Source: CAD feature listing. Evaluate the final solid. Frame: model axes, mm. Round coordinates to 2 decimals unless told otherwise and drop trailing zeros. Write each loop counter-clockwise with the first axis right and the second up, starting at its lowest first coordinate (ties: lowest second). Pieces come first, ordered by that corner, then holes. Notation, with made-up numbers: M 86.5,74 L 131.5,74 A20 ccw 131.5,101 Z; hole C 79.25,-22.5 d7. An arc over 180 degrees is marked long. Use a Markdown table: item, result.
```python
from build123d import *

# Parameters (mm, degrees)
PAD_DEPTH = 10


with BuildPart() as part:
    # Sketch → Pad (new body)
    with BuildSketch(Plane.XY):
        with BuildLine():
            Line((2.012226, 0), (22.012226, 0))
            ThreePointArc((22.012226, 0), (25.943926, 1.628563), (27.572489, 5.560263))
            Line((27.572489, 5.560263), (27.572489, 423.618953))
            ThreePointArc((46.701722, 450.938329), (32.830223, 440.294353), (27.572489, 423.618953))
            Line((46.701722, 450.938329), (760.532733, 710.751569))
            Line((760.532733, 713.751569), (760.532733, 710.751569))
            Line((24.572489, 455.938329), (760.532733, 713.751569))
            Line((24.572489, 3), (24.572489, 455.938329))
            Line((-1.804961, 3), (24.572489, 3))
            Line((-1.804961, -7), (-1.804961, 3))
            Line((21.983993, -7), (-1.804961, -7))
            Line((21.983993, -4), (21.983993, -7))
            Line((1.983993, -4), (21.983993, -4))
            ThreePointArc((0, -2.016007), (0.581098, -3.418902), (1.983993, -4))
            Line((0, -2.012226), (0, -2.016007))
            ThreePointArc((2.012226, 0), (0.589367, -0.589367), (0, -2.012226))
        make_face()
    extrude(amount=PAD_DEPTH)


solid = part.part
```
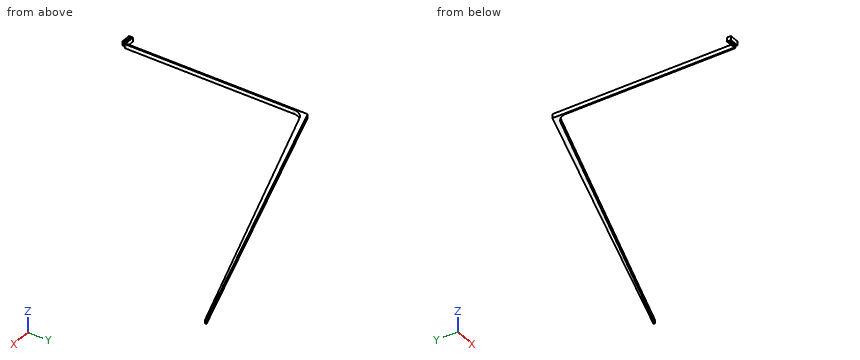
Q1. Line query: L1, parallel to X at y = 299, z = 7.25; L2, parallel to Y at x = 522.5, z = 8.75; L3, parallel to Y at x = 458, z = 3.25. Output: solid intervals per line, ascending.
Results are:
| item | result |
|---|---|
| L1 | 24.57 to 27.57 |
| L2 | 624.11 to 630.37 |
| L3 | 600.64 to 607.77 |
Q2. Section C-C on x = 332. Return loops of the section in (y, z), plus the area to 3 significant figures.
Results are:
| item | result |
|---|---|
| outline | M 554.78,0 L 563.63,0 L 563.63,10 L 554.78,10 Z |
| area | 88.5 mm^2 |
Q3. Section B-B on y = 105. Return loops of the section in (x, z).
Results are:
| item | result |
|---|---|
| outline | M 24.57,0 L 27.57,0 L 27.57,10 L 24.57,10 Z |
Q4. First-contact query: pin 1 Ø6 at (x, z) = (409.5, 1.5) entering from +Y; pin 2 Ø0.9 at (y, z) = (-5.5, 3.5) entering from +X; pin 3 Ø3 at (y, z) = (270, 4.5) entering from -X. Flat tips, straight axial feed; report the tip coordinate or a pass-through.
Results are:
| item | result |
|---|---|
| pin 1 | y = 591.83 |
| pin 2 | x = 21.98 |
| pin 3 | x = 24.57 |
